Read the model definition and answer for the solid it produces. Units are mm, in the model's axes. Coordinates: 2 decimals unless noted, no trailing zeros. Write item = value, one per line. Start each with the question number.
1) Find the intervals of material crossed by line 1 along Z through (x, y) = (80, 23); line 2 along Z through (x, y) = (148, 12.7); line 3 along Y through (x, z) = (276, -19), in increasing order. Write a range as from..to.
2) Section A-A (x = 342) is taken. Count the separate pieces of the cut face and the enclosed holes in it, plus the area to 3 significant figures.
3) Flat-ended cylindrical pins translate along their axes: pin 1 Ø5 at (x, y) = (210.5, 12.5) entering from +Z; pin 2 Ø1.4 at (x, y) = (223.5, 12) entering from -Z. Find the tip coordinate at first contact, or state that the pin passes through.
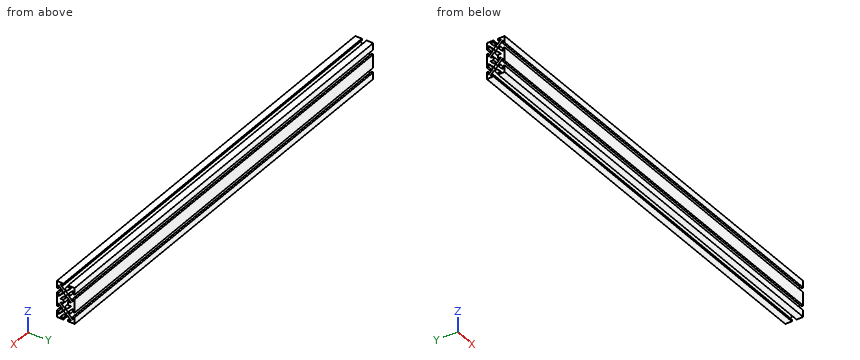
Autodesk Inventor part; units mm, degrees
ref_plane "YZ Plane" through (0, 0, 0) normal (1, 0, 0) x (0, 1, 0)
ref_plane "XZ Plane" through (0, 0, 0) normal (0, 1, 0) x (-1, 0, 0)
ref_plane "XY Plane" through (0, 0, 0) normal (0, 0, 1) x (1, 0, 0)
sketch "Sketch1" plane through (0, 0, 0) normal (1, 0, 0) x (0, 1, 0)
  line L0 (0, 0) -> (0, -9.398)
  line L1 (0, -9.398) -> (2.4765, -9.398)
  line L2 (9.398, -2.4765) -> (9.398, 0)
  line L3 (9.398, 0) -> (0, 0)
  line L4 (16.002, 0) -> (16.002, -2.4765)
  line L5 (22.9235, -9.398) -> (25.4, -9.398)
  line L6 (25.4, -9.398) -> (25.4, 0)
  line L7 (25.4, 0) -> (16.002, 0)
  line L8 (25.4, -16.002) -> (22.9235, -16.002)
  line L9 (16.002, -22.9235) -> (16.002, -25.4)
  line L10 (25.4, -25.4) -> (25.4, -16.002)
  line L11 (0, -16.002) -> (2.4765, -16.002)
  line L12 (9.398, -22.9235) -> (9.398, -25.4)
  line L13 (0, -25.4) -> (0, -16.002)
  line L14 (22.9235, -9.398) -> (22.9235, -4.953)
  line L15 (16.002, -2.4765) -> (20.447, -2.4765)
  line L16 (20.447, -2.4765) -> (15.0495, -7.874)
  line L17 (20.447, -2.4765) -> (28.0802, -2.4765) construction
  line L18 (22.9235, -4.953) -> (17.526, -10.3505)
  line L19 (22.9235, -16.002) -> (22.9235, -20.447)
  line L20 (22.9235, -20.447) -> (17.526, -15.0495)
  line L21 (16.002, -22.9235) -> (20.447, -22.9235)
  line L22 (20.447, -22.9235) -> (15.0495, -17.526)
  line L23 (2.4765, -16.002) -> (2.4765, -20.447)
  line L24 (2.4765, -20.447) -> (7.874, -15.0495)
  line L25 (9.398, -22.9235) -> (4.953, -22.9235)
  line L26 (4.953, -22.9235) -> (10.3505, -17.526)
  line L27 (9.398, -2.4765) -> (4.953, -2.4765)
  line L28 (4.953, -2.4765) -> (10.3505, -7.874)
  line L29 (2.4765, -9.398) -> (2.4765, -4.953)
  line L30 (2.4765, -4.953) -> (7.874, -10.3505)
  line L31 (10.3505, -7.874) -> (15.0495, -7.874)
  line L32 (17.526, -10.3505) -> (17.526, -15.0495)
  line L33 (10.3505, -17.526) -> (15.0495, -17.526)
  line L34 (7.874, -15.0495) -> (7.874, -10.3505)
  circle A0 centre (12.7, -12.7) radius 2.54
  line L35 (0, -50.8) -> (0, -41.402)
  line L36 (0, -41.402) -> (2.4765, -41.402)
  line L37 (9.398, -48.3235) -> (9.398, -50.8)
  line L38 (9.398, -50.8) -> (0, -50.8)
  line L39 (16.002, -50.8) -> (16.002, -48.3235)
  line L40 (22.9235, -41.402) -> (25.4, -41.402)
  line L41 (25.4, -41.402) -> (25.4, -50.8)
  line L42 (25.4, -50.8) -> (16.002, -50.8)
  line L43 (25.4, -34.798) -> (22.9235, -34.798)
  line L44 (16.002, -27.8765) -> (16.002, -25.4)
  line L45 (25.4, -25.4) -> (25.4, -34.798)
  line L46 (0, -34.798) -> (2.4765, -34.798)
  line L47 (9.398, -27.8765) -> (9.398, -25.4)
  line L48 (0, -25.4) -> (0, -34.798)
  line L49 (22.9235, -41.402) -> (22.9235, -45.847)
  line L50 (16.002, -48.3235) -> (20.447, -48.3235)
  line L51 (20.447, -48.3235) -> (15.0495, -42.926)
  line L52 (20.447, -48.3235) -> (28.0802, -48.3235) construction
  line L53 (22.9235, -45.847) -> (17.526, -40.4495)
  line L54 (22.9235, -34.798) -> (22.9235, -30.353)
  line L55 (22.9235, -30.353) -> (17.526, -35.7505)
  line L56 (16.002, -27.8765) -> (20.447, -27.8765)
  line L57 (20.447, -27.8765) -> (15.0495, -33.274)
  line L58 (2.4765, -34.798) -> (2.4765, -30.353)
  line L59 (2.4765, -30.353) -> (7.874, -35.7505)
  line L60 (9.398, -27.8765) -> (4.953, -27.8765)
  line L61 (4.953, -27.8765) -> (10.3505, -33.274)
  line L62 (9.398, -48.3235) -> (4.953, -48.3235)
  line L63 (4.953, -48.3235) -> (10.3505, -42.926)
  line L64 (2.4765, -41.402) -> (2.4765, -45.847)
  line L65 (2.4765, -45.847) -> (7.874, -40.4495)
  line L66 (10.3505, -42.926) -> (15.0495, -42.926)
  line L67 (17.526, -40.4495) -> (17.526, -35.7505)
  line L68 (10.3505, -33.274) -> (15.0495, -33.274)
  line L69 (7.874, -35.7505) -> (7.874, -40.4495)
  circle A1 centre (12.7, -38.1) radius 2.54
  dimension "d2" = 9.398
  dimension "d3" = 2.4765
  dimension "d7" = 2.4765
  dimension "d10" = 2.4765
  dimension "d11" = 25.4
  dimension "d13" = 2.4765
  dimension "d16" = 2.4765
  dimension "d17" = 9.398
  dimension "d23" = 2.4765
  dimension "d25" = 25.4
  dimension "d32" = 4.445
  dimension "d33" = 4.445
  dimension "d35" = 135
  dimension "d36" = 4.445
  dimension "d37" = 4.445
  dimension "d38" = 2.4765
  dimension "d40" = 4.445
  dimension "d41" = 4.445
  dimension "d42" = 4.445
  dimension "d43" = 4.445
  dimension "d44" = 5.08
extrude "Extrusion1" add sketch "Sketch1" along normal blind 609.6
properties part number "LatX24in1"
Answer key:
q1.line_1 = -50.8..-41.4, -34.8..-16, -9.4..0
q1.line_2 = -42.93..-40.64, -35.56..-33.27, -17.53..-15.24, -10.16..-7.87
q1.line_3 = 0..2.48, 3.92..8.88, 16.52..21.48, 22.92..25.4
q2.separate_pieces = 1
q2.enclosed_holes = 3
q2.area = 683 mm^2
q3.pin_1 = -7.52
q3.pin_2 = -42.93
